Read the model definition and answer for the solid it produces. Units are mm, in the model's axes. A direction names the side the tool comes from. Round coordinates to 2 decimals unless told otherwise and drop trailing zeros. Write each loop counter-clockwise with the first axis right and the second up, starting at its lowest first coordinate (ties: lowest second). Pieces come first, ordered by that corner, then holes.
Autodesk Inventor part; units mm, degrees
ref_plane "YZ Plane" through (0, 0, 0) normal (1, 0, 0) x (0, 1, 0)
ref_plane "XZ Plane" through (0, 0, 0) normal (0, 1, 0) x (-1, 0, 0)
ref_plane "XY Plane" through (0, 0, 0) normal (0, 0, 1) x (1, 0, 0)
sketch "Szkic1" plane through (0, 0, 0) normal (0, 1, 0) x (-1, 0, 0)
  line L0 (0, 0) -> (-11.176, 0)
  line L1 (-11.176, 0) -> (-11.176, -17.272)
  line L2 (-11.176, -17.272) -> (0, -17.272)
  line L3 (0, -17.272) -> (0, 0)
  dimension "d0" = 17.272
  dimension "d1" = 11.176
extrude "Wyciągnięcie proste1" add sketch "Szkic1" along normal blind 1.6
sketch "Szkic2" plane through (0, 1.6, 0) normal (0, 1, 0) x (1, 0, 0)
  line L0 (11.176, 0) -> (11.176, 17.272)
  line L1 (11.176, 17.272) -> (0, 17.272)
  line L2 (0, 17.272) -> (0, 0)
  line L3 (0, 0) -> (11.176, 0)
  circle A0 centre (1.016, 1.016) radius 0.55
  circle A1 centre (1.016, 16.256) radius 0.55
  circle A2 centre (10.16, 1.016) radius 0.55
  circle A3 centre (10.16, 16.256) radius 0.55
  line L4 (1.016, 1.016) -> (1.016, 16.256)
  line L5 (1.016, 16.256) -> (10.16, 16.256)
  point P0 (1.016, 8.636)
  point P1 (0, 8.636)
  point P2 (5.588, 16.256)
  point P3 (5.588, 17.272)
  dimension "d4" = 1.1
  dimension "d5" = 1.1
  dimension "d6" = 1.1
  dimension "d7" = 1.1
  dimension "d8" = 15.24
  dimension "d9" = 9.144
extrude "Wyciągnięcie proste2" cut sketch "Szkic2" against normal through all contours A0 | A3 | A1 L5 L4 | L4 L5 A1 | A2
sketch "Szkic3" plane through (0, 1.6, 0) normal (0, 1, 0) x (1, 0, 0)
  circle A0 centre (4, 7) radius 2.2361
  line L0 (7, 4) -> (9, 4)
  line L1 (9, 4) -> (9, 5)
  line L2 (9, 5) -> (7, 5)
  line L3 (7, 5) -> (7, 4)
  line L4 (7, 7) -> (9, 7)
  line L5 (9, 7) -> (9, 8)
  line L6 (9, 8) -> (7, 8)
  line L7 (7, 8) -> (7, 7)
  line L8 (7, 9.4289) -> (9, 9.4289)
  line L9 (9, 9.4289) -> (9, 10.5737)
  line L10 (9, 10.5737) -> (7, 10.5737)
  line L11 (7, 10.5737) -> (7, 9.4289)
  line L12 (2, 11) -> (6, 11)
  line L13 (6, 11) -> (6, 14)
  line L14 (6, 14) -> (2, 14)
  line L15 (2, 14) -> (2, 11)
  point P0 (0, 0)
extrude "Wyciągnięcie proste3" add sketch "Szkic3" along normal blind 1
extrude "Wyciągnięcie proste4" add sketch "Szkic3" along normal blind 2 contours A0
properties part number "MH-MINI-360"
Q1. Which of the six approach directions +Z, -Z, +X, -X, +Y, -Y give full straight-line access (tool end or side, diameter ignored) to faces 1 (the flat face through (7, 2, -10)), 2 (the flat face through (2, 2, -13)), 3 (the flat face through (8, 2, -4)), 4 (the flat face through (8, 2, -8)), 5 (the flat face through (4, 2, -11))?
Verdict:
face 1: +Z, -Z, -X, +Y
face 2: -Z, -X, +Y
face 3: +Z, +X, -X, +Y
face 4: +X, +Y
face 5: +X, -X, +Y
Q2. Section B-B (y = 1.8) is taken. Determine the outline of the cut face in (x, z).
Verdict:
outline: circle Ø4.47 at (4, -7); (2, -14) - (6, -14) - (6, -11) - (2, -11) - close; (7, -10.57) - (9, -10.57) - (9, -9.43) - (7, -9.43) - close; (7, -8) - (9, -8) - (9, -7) - (7, -7) - close; (7, -5) - (9, -5) - (9, -4) - (7, -4) - close
Q3. Section C-C (z = -11.75) is taken. Determine the outline of the cut face in (x, y).
Verdict:
outline: (0, 0) - (11.18, 0) - (11.18, 1.6) - (6, 1.6) - (6, 2.6) - (2, 2.6) - (2, 1.6) - (0, 1.6) - close
Q4. Flat-ended cylindrical pins translate along their axes: pin 1 Ø0.5 at (y, z) = (2, -7.5) entering from +X; pin 2 Ø1.1 at (y, z) = (2.5, -13) entering from +X; pin 3 Ø1.8 at (x, z) = (1.016, -16.256) entering from +Y. Find the tip coordinate at first contact, or state that the pin passes through.
Verdict:
pin 1: stops at x = 9
pin 2: stops at x = 6
pin 3: stops at y = 1.6
Q5. Straight lines are drawn through the part: probe 1 along Z at (x, y) = (10.16, 1); probe 2 along Z at (x, y) = (8.5, 1.9); probe 3 along Y at (x, z) = (9.25, -13.25). For each, find the intervals that lie inside material, in ascending order.
Verdict:
probe 1: z = -17.27 to -16.81, -15.71 to -1.57, -0.47 to 0
probe 2: z = -10.57 to -9.43, -8 to -7, -5 to -4
probe 3: y = 0 to 1.6
Q6. Section A-A (x = 10.16) is taken. Determine the outline of the cut face in (y, z).
Verdict:
outline: (0, -17.27) - (1.6, -17.27) - (1.6, -16.81) - (0, -16.81) - close; (0, -15.71) - (1.6, -15.71) - (1.6, -1.57) - (0, -1.57) - close; (0, -0.47) - (1.6, -0.47) - (1.6, 0) - (0, 0) - close
Q7. Section D-D (x = 4) is taken. Determine the outline of the cut face in (y, z).
Verdict:
outline: (0, -17.27) - (1.6, -17.27) - (1.6, -14) - (2.6, -14) - (2.6, -11) - (1.6, -11) - (1.6, -9.24) - (3.6, -9.24) - (3.6, -4.76) - (1.6, -4.76) - (1.6, 0) - (0, 0) - close
